Work out the finished part from the listing and answer in its coordinate system (mm). Face numbers are marked on the shaded views. A direction names the side the tool comes from. Coordinates: 2 decimals unless noted, no trailing zeros. Loops run counter-clockwise (first coordinate to the right, second up) from the corner with the lowest first, then second, coordinate; pieces in that order, holes last. Notation, with made-up numbers: (77.5, -23) - (114.5, -23) arc R4 cw to (114.5, -19) - close; hole circle Ø5 at (42.5, 10). An arc over 180 degrees is marked (long way). Write each question's results on one line, items separated by ' | '. Start each with the question number.
1. Each of these flat-tipped pins is pushed along its axis until it touches: P1, Ø1, axis at x = 0, y = -0.5, coming from the +Z side; P2, Ø1, axis at x = -2, y = -2, coming from the +Z side; P3, Ø0.6, axis at x = -1.5, y = -0.5, coming from the -Z side. Where does it stop, or does it pass through?
2. A cutting plane is placed at B-B on z = -0.5. Determine the outline of the cut face in (x, y), then the cut area to 3 significant figures.
3. A cutting plane is placed at C-C on y = -2.45. Determine the outline of the cut face in (x, z).
4. Which of the six approach directions +Z, -Z, +X, -X, +Y, -Y give full straight-line access (tool end or side, diameter ignored) to the marked faces 4 and 5?
5. Determine the mould class of the marked faces 1, 2 and 3 for opening direction Z: released by +Z, released by -Z, zero draft, split by the parting line, or undercut.
6. A cutting plane is placed at D-D on x = -2.5. Determine the outline of the cut face in (y, z), then the cut area to 3 significant figures.
7. A cutting plane is placed at A-A on x = 0. Determine the outline of the cut face in (y, z).
8. Find the intervals of material crossed by line 1 along Z through (x, y) = (0, -0.95); line 2 along Z through (x, y) = (0, -1.8); line 3 along X through (y, z) = (-3.5, -0.75), in increasing order. Write a range as [from, to].
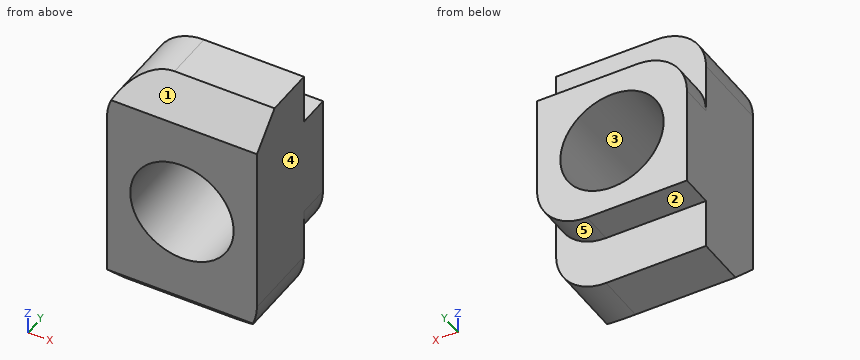
from build123d import *

# Parameters (mm, degrees)
BOSS_EXTRUDE1_DEPTH = 3
FILLET1_R           = 2
TAP1_D              = 4.134


with BuildPart() as part:
    # Sketch1 → Boss-Extrude1 (new body, symmetric)
    with BuildSketch(Plane(origin=(0, 0, 0), x_dir=(0, 0, -1), z_dir=(1, 0, 0))):
        Polygon((-3, 0), (3, 0), (3, -1.3), (5, -1.3), (5, -3.3), (3.8, -4.5), (-3.8, -4.5), (-5, -3.3), (-5, -1.3), (-3, -1.3), align=None)
    extrude(amount=BOSS_EXTRUDE1_DEPTH, both=True)

    # Fillet1
    fillet1_edges = [part.edges().sort_by_distance(p)[0] for p in [
        (3, -2.3, -5),
        (-3, -2.3, 5),
        (3, -0.65, -3),
        (-3, -0.65, 3),
    ]]
    fillet(fillet1_edges, radius=FILLET1_R)

    # Tap1 (through all)
    with Locations(Plane(origin=(0, 0, 0), x_dir=(1, 0, 0), z_dir=(0, 1, 0))):
        with Locations((0, 0)):
            Hole(TAP1_D / 2)


solid = part.part
Values:
1) P1: z = 3 | P2: z = 4.94 | P3: z = -3
2) outline: (-3, -4.5) - (-2.01, -4.5) - (-2.01, 0) - (-3, 0) - close; (2.01, -4.5) - (3, -4.5) - (3, 0) - (2.01, 0) - close | area: 8.95 mm^2
3) outline: (-3, -5) - (1, -5) arc R2 ccw to (3, -3) - (3, 5) - (-1, 5) arc R2 ccw to (-3, 3) - close; hole circle Ø4.13 at (0, 0)
4) face 4: +Z, -Z, +X, +Y, -Y | face 5: -Z, +X, +Y
5) face 1: released by +Z | face 2: released by -Z | face 3: undercut
6) outline: (-4.5, -3.8) - (-3.3, -5) - (-1.3, -5) - (-1.3, -3) - (0, -3) - (0, 2.32) - (-1.3, 2.32) - (-1.3, 4.32) - (-3.98, 4.32) - (-4.5, 3.8) - close | area: 35.9 mm^2
7) outline: (-4.5, -3.8) - (-3.3, -5) - (-1.3, -5) - (-1.3, -3) - (0, -3) - (0, -2.07) - (-4.5, -2.07) - close; (-4.5, 2.07) - (0, 2.07) - (0, 3) - (-1.3, 3) - (-1.3, 5) - (-3.3, 5) - (-4.5, 3.8) - close
8) line 1: [-3, -2.07], [2.07, 3] | line 2: [-5, -2.07], [2.07, 5] | line 3: [-3, -1.93], [1.93, 3]
